The listing builds one solid part. Answer for the finished solid, in the listing's coordinates (mm). Face numbers are marked on the shaded views. A direction names the side the tool comes from. Coordinates: 2 decimals unless noted, no trailing zeros. Loops run counter-clockwise (first coordinate to the right, second up) from the corner with the lowest first, then second, coordinate; pieces in that order, holes last. Notation, with made-up numbers: (85, 81) - (134, 81) arc R11 ccw to (134, 91) - close; hole circle Ø7 at (11.5, 66). An arc over 180 degrees is marked (long way). Return JSON: item names as keys, results as strings. Group by question number.
1. Find the intervals of material crossed by line 1 along X through (y, z) = (30, -33); line 2 along Z through (x, y) = (6, 406); line 3 along Y through (x, z) = (2, 57), in increasing order.
2. The mould has two halves that part along Z. Classify the marked faces 1, 2 and 3: pulls with the +Z half, pulls with the -Z half, needs draft (parallel to the pull), parting line crosses it, or undercut.
3. Each of these flat-tipped pins is pushed along its axis until it touches: P1, Ø19.5, axis at x = 0, y = 430, coming from the +Z side; P2, Ø12, axis at x = -1.5, z = -35.5, coming from the +Y side; P3, Ø12, axis at x = 0, y = 430, coming from the +Z side. Where does it stop, or does it pass through?
4. Which of the six approach directions +Z, -Z, +X, -X, +Y, -Y give full straight-line access (tool end or side, diameter ignored) to the marked faces 4 and 5?
5. Section B-B (z = 12.5) is taken. Write down the section's boundary in (x, y), and give its area (3 significant figures).
6. Section A-A (x = 0) is taken. Write down the section's boundary in (y, z).
Autodesk Inventor part; units mm, degrees
ref_plane "YZ Plane" through (0, 0, 0) normal (1, 0, 0) x (0, 1, 0)
ref_plane "XZ Plane" through (0, 0, 0) normal (0, 1, 0) x (-1, 0, 0)
ref_plane "XY Plane" through (0, 0, 0) normal (0, 0, 1) x (1, 0, 0)
sketch "Boceto1" plane through (0, 0, 0) normal (0, 1, 0) x (-1, 0, 0)
  line L0 (-25, 65) -> (25, 65)
  line L1 (25, 65) -> (25, -65)
  line L2 (25, -65) -> (-25, -65)
  line L3 (-25, -65) -> (-25, 65)
  line L4 (-25, 65) -> (25, -65) construction
  line L5 (25, 65) -> (-25, -65) construction
  point P0 (0, 0)
  dimension "d0" = 50
  dimension "d1" = 130
extrude "Extrusión1" add sketch "Boceto1" along normal blind 400
sketch "Boceto2" plane through (-25, 0, 65) normal (0, 0, 1) x (1, 0, 0)
  line L0 (0, 400) -> (50, 400)
  line L1 (0, 400) -> (0, 430)
  line L2 (50, 400) -> (50, 430)
  arc A0 (50, 430) -> (0, 430) centre (25, 430) ccw
  circle A1 centre (25, 430) radius 7.5
  point P0 (25, 0)
  dimension "d4" = 30
  dimension "d5" = 30
  dimension "d6" = 15
extrude "Extrusión2" add sketch "Boceto2" against normal blind 10
sketch "Boceto3" plane through (25, 0, -65) normal (0, 0, -1) x (-1, 0, 0)
  arc A0 (50, 430) -> (0, 430) centre (25, 430) ccw
  circle A1 centre (25, 430) radius 7.5
  line L0 (50, 400) -> (50, 430)
  line L1 (0, 400) -> (50, 400)
  line L2 (0, 430) -> (0, 400)
  point P0 (25, 0)
extrude "Extrusión3" add sketch "Boceto3" against normal blind 10
sketch "Boceto4" plane through (25, 0, -65) normal (0, 0, -1) x (-1, 0, 0)
  line L0 (25, 0) -> (25, 30)
  circle A0 centre (25, 30) radius 7.5
  dimension "d11" = 30
  dimension "d12" = 15
extrude "Extrusión4" cut sketch "Boceto4" against normal up to next
properties part number "brazo 1"
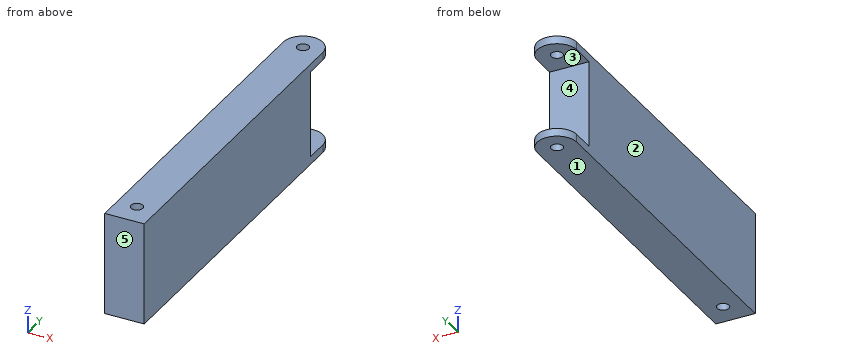
The answers:
{
 "1": {"line 1": "x = -25 to -7.5, 7.5 to 25", "line 2": "z = -65 to -55, 55 to 65", "line 3": "y = 0 to 22.77, 37.23 to 422.77, 437.23 to 454.92"},
 "2": {"face 1": "pulls with the -Z half", "face 2": "needs draft", "face 3": "undercut"},
 "3": {"P1": "stops at z = 65", "P2": "stops at y = 400", "P3": "passes through"},
 "4": {"face 4": "+X, -X, +Y", "face 5": "+Z, -Z, +X, -X, -Y"},
 "5": {"outline": "(-25, 0) - (25, 0) - (25, 400) - (-25, 400) - close; hole circle Ø15 at (0, 30)", "area": "19,800 mm2"},
 "6": {"outline": "(0, -65) - (22.5, -65) - (22.5, 65) - (0, 65) - close; (37.5, -65) - (422.5, -65) - (422.5, -55) - (400, -55) - (400, 55) - (422.5, 55) - (422.5, 65) - (37.5, 65) - close; (437.5, -65) - (455, -65) - (455, -55) - (437.5, -55) - close; (437.5, 55) - (455, 55) - (455, 65) - (437.5, 65) - close"}
}
